The model under review builds one solid part; all positions refer to its coordinate system, in mm. A direction names the side the tool comes from. Give positions to 0.01 mm unless a question says otherwise; leave off trailing zeros. Write each loop counter-clockwise with the first axis right and the second up, starting at its lowest first coordinate (ties: lowest second). Pieces come first, ordered by that corner, then holes. Notation, with made-up numbers: (-27.5, 58) - (24.5, 58) arc R24 cw to (24.5, 79) - close; hole circle Ø10 at (-30.75, 59). An arc over 180 degrees is marked (long way). Write item = value, one per line.
```python
from build123d import *

# Parameters (mm, degrees)
CORTAR_EXTRUIR1_REACH = 70.338
CROQUIS2_R            = 12


with BuildPart() as part:
    # Croquis1 → Revolución1 (revolve)
    with BuildSketch(Plane.XY, mode=Mode.PRIVATE) as revoluci_n1_sk:
        Polygon((7.730917784, 46.314331723), (7.730917784, 12.628663446), (22.730917784, 12.628663446), (27.730917784, 24.989291465), (40.730917784, 24.989291465), (42.730917784, 16.471497585), (45.730917784, 16.471497585), (45.730917784, 42.471497585), (42.730917784, 42.471497585), (40.730917784, 33.953703704), (27.730917784, 33.953703704), (22.730917784, 46.314331723), align=None)
    revolve(revoluci_n1_sk.sketch.rotate(Axis((7.730917784, 46.314331723, 0), (0, -1, 0)), 90), axis=Axis((7.730917784, 46.314331723, 0), (0, -1, 0)))

    # Croquis2 → Cortar-Extruir1 (cut, up to next)
    with BuildSketch(Plane(origin=(0, 46.314331723, 0), x_dir=(1, 0, 0), z_dir=(0, 1, 0)), mode=Mode.PRIVATE) as cortar_extruir1_sk1:
        with Locations(Location((7.730917784, 0, 0), (0, 0, 270))):
            Circle(CROQUIS2_R)
    cortar_extruir1_tool1 = extrude(cortar_extruir1_sk1.sketch, amount=-CORTAR_EXTRUIR1_REACH, mode=Mode.PRIVATE) & part.part
    add(cortar_extruir1_tool1.solids().sort_by_distance((7.730918, 46.314332, 0))[0], mode=Mode.SUBTRACT)


solid = part.part
```
1. Take a section at A-A on z = 0. Give the boundary of the cut face in (x, y), and give its area (3 significant figures).
Findings below:
outline = (-30.27, 16.47) - (-27.27, 16.47) - (-25.27, 24.99) - (-12.27, 24.99) - (-7.27, 12.63) - (-4.27, 12.63) - (-4.27, 46.31) - (-7.27, 46.31) - (-12.27, 33.95) - (-25.27, 33.95) - (-27.27, 42.47) - (-30.27, 42.47) - close; (19.73, 12.63) - (22.73, 12.63) - (27.73, 24.99) - (40.73, 24.99) - (42.73, 16.47) - (45.73, 16.47) - (45.73, 42.47) - (42.73, 42.47) - (40.73, 33.95) - (27.73, 33.95) - (22.73, 46.31) - (19.73, 46.31) - close
area = 874 mm²
2. Draft analysis for pull direction X (two halves, no side actions). For faces 1 (the conical face through (40.041, 34.367, -7.175)), 2 (the flat face through (39, 42.471, 17)), 3 (the cylindrical face through (44.827, 29.653, -8.238)), state which applies: +X half, -X half, draft (parallel to the pull), parting line (faces both ways), or undercut.
Findings below:
face_1 = undercut
face_2 = draft
face_3 = parting line
3. Take a section at B-B on y = 20. Give the boundary of the cut face in (x, z), and give its area (3 significant figures).
Findings below:
outline = circle Ø76 at (7.73, 0); circle Ø35.96 at (7.73, 0); hole circle Ø68.34 at (7.73, 0); hole circle Ø24 at (7.73, 0)
area = 1,430 mm²
4. Take a section at D-D on y = 37.5. Give the boundary of the cut face in (x, z), and give its area (3 significant figures).
Findings below:
outline = circle Ø76 at (7.73, 0); circle Ø37.13 at (7.73, 0); hole circle Ø67.67 at (7.73, 0); hole circle Ø24 at (7.73, 0)
area = 1,570 mm²
5. Take a section at C-C on y = 30.5. Give the boundary of the cut face in (x, z).
Findings below:
outline = circle Ø76 at (7.73, 0); hole circle Ø24 at (7.73, 0)
6. Machinability: for faces 4 (the flat face through (29, 33.954, 0)), 5 (the flat face through (-5, 46.314, 0)), 6 (the flat face through (39, 16.471, -17)), which of the approach directions +Z, -Z, +X, -X, +Y, -Y give a long, thin tool a straight path to every point of the face, cutting with its end or side? Answer none if there is none.
Findings below:
face_4 = +Y
face_5 = +Z, -Z, +X, -X, +Y
face_6 = -Y
7. For line 1 (X direction, y = 33, z = 0); line 2 (Z direction, x = 22.5, y = 34.5); line 3 (X direction, y = 21, z = 0), list the stretches that pass through material, from the lowest coordinate up. Write a range as from..to.
Findings below:
line_1 = -30.27..-4.27, 19.73..45.73
line_2 = -35.01..-29.65, -13.16..13.16, 29.65..35.01
line_3 = -30.27..-26.21, -10.66..-4.27, 19.73..26.12, 41.67..45.73
8. Insertion check: P1, Ø10, axis at x = 6, y = 18, coming from the -Z side; P2, Ø4, axis at x = -9, y = 22, coming from the -Z side; P3, Ø5, axis at y = 24.5, z = 20, coming from the +X side; P4, Ø3, axis at x = -2.5, y = 20, coming from the +Z side. Each pin has a flat end and moves straight along its axis. Give the tip position at first contact, or say it passes through.
Findings below:
P1 = -38
P2 = -35.03
P3 = 41.46
P4 = 36.98
